The model under review builds one solid part; all positions refer to its coordinate system, in mm. A direction names the side the tool comes from. Coordinates: 2 decimals unless noted, no trailing zeros. Order: outer loops, then holes, each group sorted by start corner. A loop starts at its lowest first (then second) coordinate and runs counter-clockwise, first axis right, second up. Notation, with made-up numbers: M 6,-32.5 L 27,-32.5 A29 cw 27,-1.5 Z; hole C 85,19 d9. An arc over 180 degrees is marked long. Write each question's results on one line, items separated by ' | '.
from build123d import *

# Parameters (mm, degrees)
SKETCH_1_R          = 1.8
SKETCH_1_R_2        = 5
EXTRUDE_1_DEPTH     = 3
EXTRUDE_2_DEPTH     = 2.2
SKETCH_3_R          = 5
CUT_EXTRUDE_1_DEPTH = 2.2
EXTRUDE_4_DEPTH     = 2.2
EXTRUDE_5_DEPTH     = 2.2


with BuildPart() as part:
    # 草图1 → 凸台-拉伸1 (new body)
    with BuildSketch(Plane(origin=(0, 0, 0), x_dir=(1, 0, 0), z_dir=(0, 1, 0))):
        with BuildLine():
            Line((20, -3.872983346), (20, -15))
            ThreePointArc((20, -15), (18.535533906, -18.535533906), (15, -20))
            Line((15, -20), (-15, -20))
            ThreePointArc((-15, -20), (-18.535533906, -18.535533906), (-20, -15))
            Line((-20, -15), (-20, -3.872983346))
            ThreePointArc((-20, -3.872983346), (-14, 0), (-20, 3.872983346))
            Line((-20, 3.872983346), (-20, 15))
            ThreePointArc((-20, 15), (-18.535533906, 18.535533906), (-15, 20))
            Line((-15, 20), (15, 20))
            ThreePointArc((15, 20), (18.535533906, 18.535533906), (20, 15))
            Line((20, 15), (20, 3.872983346))
            ThreePointArc((20, 3.872983346), (14, 0), (20, -3.872983346))
        make_face()
        with Locations(Location((-15.5, 15.5, 0), (0, 0, 270))):
            Circle(SKETCH_1_R, mode=Mode.SUBTRACT)
        with Locations(Location((15.5, 15.5, 0), (0, 0, 270))):
            Circle(SKETCH_1_R, mode=Mode.SUBTRACT)
        with Locations(Location((-15.5, -15.5, 0), (0, 0, 270))):
            Circle(SKETCH_1_R, mode=Mode.SUBTRACT)
        with Locations(Location((15.5, -15.5, 0), (0, 0, 270))):
            Circle(SKETCH_1_R, mode=Mode.SUBTRACT)
        with Locations(Location((0, 0, 0), (0, 0, 270))):
            Circle(SKETCH_1_R_2, mode=Mode.SUBTRACT)
    extrude(amount=EXTRUDE_1_DEPTH)

    # 草图2 → 凸台-拉伸2 (add)
    with BuildSketch(Plane(origin=(0, 3, 0), x_dir=(1, 0, 0), z_dir=(0, 1, 0))):
        with BuildLine():
            Line((-20, 3.872983346), (-7.512267775, 11.81379841))
            ThreePointArc((-7.512267775, 11.81379841), (0, 14), (7.512267775, 11.81379841))
            Line((7.512267775, 11.81379841), (20, 3.872983346))
            Line((20, 3.872983346), (20, 1.333229163))
            ThreePointArc((20, 1.333229163), (16.05, 0), (20, -1.333229163))
            Line((20, -1.333229163), (20, -3.872983346))
            Line((20, -3.872983346), (7.512267775, -11.81379841))
            ThreePointArc((7.512267775, -11.81379841), (0, -14), (-7.512267775, -11.81379841))
            Line((-7.512267775, -11.81379841), (-20, -3.872983346))
            Line((-20, -3.872983346), (-20, -1.333229163))
            ThreePointArc((-20, -1.333229163), (-16.05, 0), (-20, 1.333229163))
            Line((-20, 1.333229163), (-20, 3.872983346))
        make_face()
    extrude(amount=EXTRUDE_2_DEPTH)

    # 草图3 → 切除-拉伸1 (cut)
    with BuildSketch(Plane.XZ.offset(-3)):
        with Locations(Location((0, 0, 0), (0, 0, 270))):
            Circle(SKETCH_3_R)
    extrude(amount=-CUT_EXTRUDE_1_DEPTH, mode=Mode.SUBTRACT)

    # 草图4 → 凸台-拉伸4 (add)
    with BuildSketch(Plane.XZ.offset(-3)):
        with BuildLine():
            Line((20, 3.872983346), (20, 1.333229163))
            ThreePointArc((20, 1.333229163), (20.45, 0), (20, -1.333229163))
            Line((20, -1.333229163), (20, -3.872983346))
            ThreePointArc((20, -3.872983346), (22.5, 0), (20, 3.872983346))
        make_face()
    extrude(amount=-EXTRUDE_4_DEPTH)

    # 草图5 → 凸台-拉伸5 (add)
    with BuildSketch(Plane.XZ.offset(-3)):
        with BuildLine():
            Line((-20, 3.872983346), (-20, 1.333229163))
            ThreePointArc((-20, 1.333229163), (-20.45, 0), (-20, -1.333229163))
            Line((-20, -1.333229163), (-20, -3.872983346))
            ThreePointArc((-20, -3.872983346), (-22.5, 0), (-20, 3.872983346))
        make_face()
    extrude(amount=-EXTRUDE_5_DEPTH)


solid = part.part
1) Take a section at B-B on y = 2. State the section outline as (x, z) points, plus the area to 3 significant figures.
Solutions:
outline: M -20,-15 A5 ccw -15,-20 L 15,-20 A5 ccw 20,-15 L 20,-3.87 A4.25 cw long 20,3.87 L 20,15 A5 ccw 15,20 L -15,20 A5 ccw -20,15 L -20,3.87 A4.25 cw long -20,-3.87 Z; hole C -15.5,-15.5 d3.6; hole C -15.5,15.5 d3.6; hole C 0,0 d10; hole C 15.5,-15.5 d3.6; hole C 15.5,15.5 d3.6 | area: 1,370 mm2
2) For faces 1 (the flat face through (0, 3, -16)), 2 (the cylindrical face through (-14, 1, 0)), 3 (the flat face through (5.3, 5.2, 0.2)), 4 (the flat face through (13.67, 4.08, -7.9)), 5 (the cylindrical face through (19, 1, 18)), list the 3-axis set-ups (+Z, -Z, +X, -X, +Y, -Y) from which the entire face can be reached by the end or side of a thin tool; tool diameter is ignored.
Solutions:
face 1: -Z, +Y | face 2: -Y | face 3: +Z, -Z, +X, -X, +Y | face 4: -Z, +X, +Y | face 5: +Z, +X, +Y, -Y
3) For pin 1 (3 mm diameter, centred on x = -15.5, z = 15.5, fed in from +Y); pin 2 (2.5 mm diameter, centred on x = 20, z = -1, fed in from -Y); pin 3 (1 mm diameter, centred on y = 2, z = 13.5, fed in from +X); pin 4 (1.5 mm diameter, centred on y = 1.5, z = 8, fed in from -X), all flat-tipped, find the tip position at first contact; note any pin that passes through.
Solutions:
pin 1: through | pin 2: y = 3 | pin 3: x = 20 | pin 4: x = -20
4) The part is to be moulded in two halves that separate along Z. For faces 6 (the flat face through (-4, 0, -5)), 7 (the cylindrical face through (-18, 1, 19)), 8 (the cylindrical face through (-13.982, 1.479, 16.468)), say which applies: pulls with the +Z half, pulls with the -Z half, needs draft (parallel to the pull), parting line crosses it, or undercut.
Solutions:
face 6: needs draft | face 7: pulls with the +Z half | face 8: undercut
5) Take a section at D-D on y = 4.65. State the section outline as (x, z) points.
Solutions:
outline: M -20,-3.87 L -7.51,-11.81 A14 ccw 7.51,-11.81 L 20,-3.87 A4.25 ccw 20,3.87 L 7.51,11.81 A14 ccw -7.51,11.81 L -20,3.87 A4.25 ccw Z; hole C -18.25,0 d4.4; hole C 0,0 d10; hole C 18.25,0 d4.4
6) Take a section at A-A on x = 0. State the section outline as (y, z) points, plus the area to 3 significant figures.
Solutions:
outline: M 0,-20 L 3,-20 L 3,-14 L 5.2,-14 L 5.2,-5 L 0,-5 Z; M 0,5 L 5.2,5 L 5.2,14 L 3,14 L 3,20 L 0,20 Z | area: 130 mm2
7) Take a section at C-C on z = 0. State the section outline as (x, y) points, plus the area to 3 significant figures.
Solutions:
outline: M -22.5,3 L -20.45,3 L -20.45,5.2 L -22.5,5.2 Z; M -16.05,3 L -14,3 L -14,0 L -5,0 L -5,5.2 L -16.05,5.2 Z; M 5,0 L 14,0 L 14,3 L 16.05,3 L 16.05,5.2 L 5,5.2 Z; M 20.45,3 L 22.5,3 L 22.5,5.2 L 20.45,5.2 Z | area: 112 mm2
8) To check wall thickness, follow line 1 along X through (y, z) = (1.15, -15.5); line 2 along X through (y, z) = (4.15, -2); line 3 along Y through (x, z) = (17.5, 6.5). State the ranges of each line that lie inside material, in increasing order.
Solutions:
line 1: -19.97 to -17.3, -13.7 to 13.7, 17.3 to 19.97 | line 2: -22 to -19.17, -17.33 to -4.58, 4.58 to 17.33, 19.17 to 22 | line 3: 0 to 3
